Job drawing, mm, ordinate dimensions from the low corner. One solid piece. A direction names the side the tool comes from. Give positions to 0.01 mm unless a question says otherwise; leave off trailing zeros. Order: outer loops, then holes, each group sorted by start corner. A loop starts at its lowest first (then second) coordinate and runs counter-clockwise, first axis right, second up. Notation, with made-up numbers: M -6.5,12.25 L 33.5,12.25 A17 cw 33.5,19.25 Z; hole C 32,23 d8. An arc over 180 degrees is marked long. Put each result on its own line as item: value. Start each with the question number.
1) Two-plate mould, pull along X, no slides. Class the marked faces 4 and 5: released by +X, released by -X, zero draft, split by the parting line, or undercut.
2) Pin check, flat tips, straight feed: pin 1 (0.9 mm diameter, centred on x = 63, z = 1, fed in from +Y); pin 2 (6 mm diameter, centred on x = 46, y = 10, fed in from +Z); pin 3 (1 mm diameter, centred on y = 10.5, z = 3.5, fed in from -X). Stop position of each tip, or through.
3) Cut at B-B (z = 5.5). Write the cut outline in (x, y).
4) Tool access for the marked faces 1, 2 and 3: list every direction of +Z, -Z, +X, -X, +Y, -Y with a clear straight run to the whole face (end or side of a thin tool).
5) Drill centre lines: line 1 (X direction, y = 19, z = 1.65); line 2 (Y direction, x = 34.5, z = 3.5); line 3 (X direction, y = 28.5, z = 4.5). Where is each one in solid material? Low to high. Write a range as [from, to].
6) Cut at A-A (x = 5). Write the cut outline in (y, z), and give its area (3 significant figures).
7) Cut at D-D (x = 50.5). Write the cut outline in (y, z), and give its area (3 significant figures).
8) Cut at C-C (z = 2). Write the cut outline in (x, y).
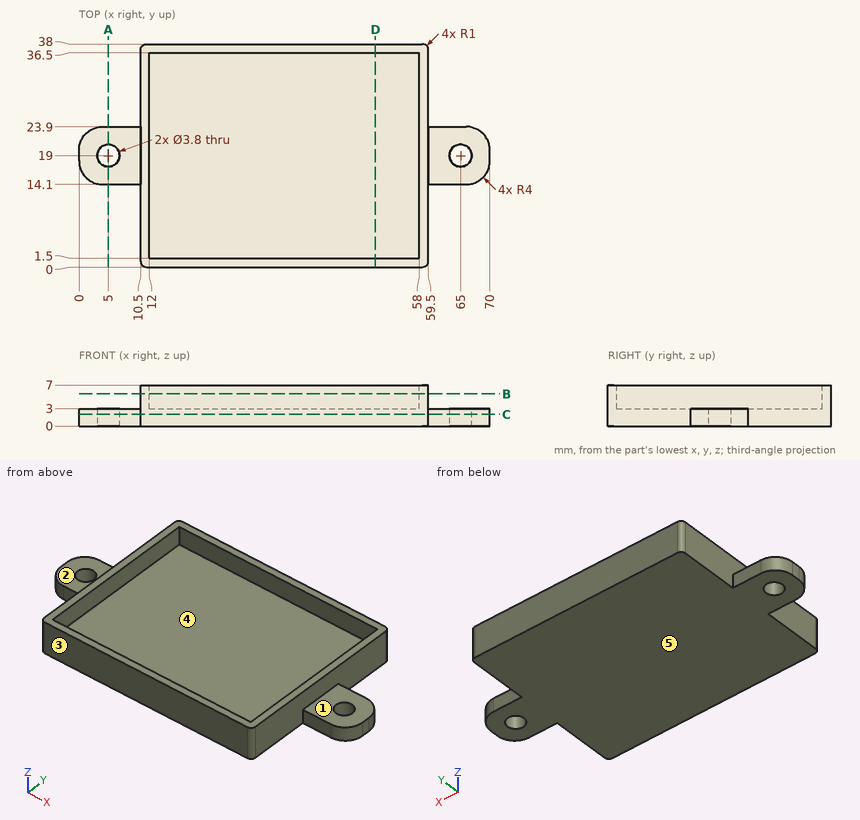
Solution:
1. face 4: undercut
1. face 5: zero draft
2. pin 1: y = 23.9
2. pin 2: z = 3
2. pin 3: x = 10.5
3. outline: M 10.5,1 A1 ccw 11.5,0 L 58.5,0 A1 ccw 59.5,1 L 59.5,37 A1 ccw 58.5,38 L 11.5,38 A1 ccw 10.5,37 Z; hole M 12,1.5 L 58,1.5 L 58,36.5 L 12,36.5 Z
4. face 1: +Z, +X, +Y, -Y
4. face 2: +Z, -X, +Y, -Y
4. face 3: +Z, -Z, +X, -X, -Y
5. line 1: [0, 3.1], [6.9, 63.1], [66.9, 70]
5. line 2: [0, 1.5], [36.5, 38]
5. line 3: [10.5, 12], [58, 59.5]
6. outline: M 14.1,0 L 17.1,0 L 17.1,3 L 14.1,3 Z; M 20.9,0 L 23.9,0 L 23.9,3 L 20.9,3 Z
6. area: 18.0 mm²
7. outline: M 0,0 L 38,0 L 38,7 L 36.5,7 L 36.5,3 L 1.5,3 L 1.5,7 L 0,7 Z
7. area: 126 mm²
8. outline: M 0,18.1 A4 ccw 4,14.1 L 10.5,14.1 L 10.5,1 A1 ccw 11.5,0 L 58.5,0 A1 ccw 59.5,1 L 59.5,14.1 L 66,14.1 A4 ccw 70,18.1 L 70,19.9 A4 ccw 66,23.9 L 59.5,23.9 L 59.5,37 A1 ccw 58.5,38 L 11.5,38 A1 ccw 10.5,37 L 10.5,23.9 L 4,23.9 A4 ccw 0,19.9 Z; hole C 5,19 d3.8; hole C 65,19 d3.8
